Autodesk Inventor part; units mm, degrees
ref_plane "YZ Plane" through (0, 0, 0) normal (1, 0, 0) x (0, 1, 0)
ref_plane "XZ Plane" through (0, 0, 0) normal (0, 1, 0) x (-1, 0, 0)
ref_plane "XY Plane" through (0, 0, 0) normal (0, 0, 1) x (1, 0, 0)
sketch "Sketch1" plane through (0, 0, 0) normal (0, 0, 1) x (1, 0, 0)
  line L0 (0, 0) -> (457.2, 0)
  line L1 (457.2, 0) -> (457.2, 457.2)
  line L2 (457.2, 457.2) -> (0, 457.2)
  line L3 (0, 457.2) -> (0, 0)
  dimension "d0" = 457.2
  dimension "d1" = 457.2
extrude "Extrusion1" add sketch "Sketch1" along normal blind 25.4
sketch "Sketch2" plane through (0, 0, 0) normal (-1, 0, 0) x (0, 0, 1)
  line L0 (0, 457.2) -> (25.4, 457.2)
  line L1 (0, 457.2) -> (0, 304.8)
  line L2 (0, 0) -> (0, 457.2)
  line L3 (25.4, 0) -> (25.4, 457.2)
  line L4 (0, 304.8) -> (25.4, 457.2)
  dimension "d4" = 152.4
extrude "Extrusion2" cut sketch "Sketch2" against normal blind 457.2
sketch "Sketch3" plane through (0, 0, 0) normal (-1, 0, 0) x (0, 0, 1)
  line L0 (25.4, 457.2) -> (25.4, 0)
  line L1 (25.4, 457.2) -> (0, 457.2)
  line L2 (0, 304.8) -> (0, 0)
  line L3 (0, 457.2) -> (0, 304.8)
  line L4 (0, 304.8) -> (25.4, 457.2)
extrude "Extrusion3" add sketch "Sketch3" against normal blind 152.4
sketch "Sketch4" plane through (457.2, 0, 25.4) normal (1, 0, 0) x (0, 0, -1)
  line L0 (0, 0) -> (0, 457.2)
  line L1 (0, 457.2) -> (25.4, 457.2)
  line L2 (25.4, 304.8) -> (0, 457.2)
  line L3 (25.4, 457.2) -> (25.4, 304.8)
  line L4 (25.4, 304.8) -> (0, 457.2)
  point P0 (25.4, 0)
extrude "Extrusion4" add sketch "Sketch4" against normal blind 152.4
sketch "Sketch5" plane through (0, 0, 0) normal (0, -1, 0) x (1, 0, 0)
  line L0 (304.8, 25.4) -> (152.4, 25.4)
  line L1 (304.8, 25.4) -> (152.4, 25.4)
  line L2 (152.4, 25.4) -> (152.4, 0)
  line L3 (152.4, 0) -> (304.8, 0)
  line L4 (304.8, 0) -> (304.8, 25.4)
  point P0 (0, 0)
extrude "Extrusion5" cut sketch "Sketch5" against normal blind 304.8
properties part number "BackLiftProtoPart3"
For this review, take the finished solid that the model builds, in its own axes (mm). A direction names the side the tool comes from. Round coordinates to 2 decimals unless told otherwise and drop trailing zeros. Write each loop counter-clockwise with the first axis right and the second up, starting at its lowest first coordinate (ties: lowest second). Pieces come first, ordered by that corner, then holes.
1) Take a section at B-B on z = 7.25. Give the boundary of the cut face in (x, y).
Answer below:
outline: (0, 0) - (152.4, 0) - (152.4, 304.8) - (304.8, 304.8) - (304.8, 0) - (457.2, 0) - (457.2, 457.2) - (304.8, 457.2) - (304.8, 348.3) - (152.4, 348.3) - (152.4, 457.2) - (0, 457.2) - close
2) Take a section at A-A on y = 36.5. Give the boundary of the cut face in (x, z), then the cut area to 3 significant figures.
Answer below:
outline: (0, 0) - (152.4, 0) - (152.4, 25.4) - (0, 25.4) - close; (304.8, 0) - (457.2, 0) - (457.2, 25.4) - (304.8, 25.4) - close
area: 7,740 mm2
3) Machinability: for faces 1 (the face through (228, 304.8, 13)), 2 (the face through (227.53, 379.93, 12.52)), 3 (the face through (75, 0, 13)), which of the approach directions +Z, -Z, +X, -X, +Y, -Y give a long, thin tool a straight path to every point of the face, cutting with its end or side? Answer none if there is none.
Answer below:
face 1: +Z, -Z, -Y
face 2: -Z, +Y
face 3: +Z, -Z, +X, -X, -Y
4) Take a section at C-C on x = 172. Give the boundary of the cut face in (y, z).
Answer below:
outline: (304.8, 0) - (457.2, 25.4) - (304.8, 25.4) - close
5) Insertion check: pin 1 Ø12 at (y, z) = (197.5, 21.5) entering from -X; pin 2 Ø12.5 at (x, z) = (232.5, 17.5) entering from -Y. Each pin has a flat end and moves straight along its axis. Give the tip position at first contact, or say it passes through.
Answer below:
pin 1: stops at x = 0
pin 2: stops at y = 304.8
6) Mouldability with a two-part tool opening along X and no side actions: class faces 4 (the face through (457.2, 232, 13)), 5 (the face through (304.8, 150, 13)), 6 (the face through (382, 457.2, 13)) as +X half, -X half, draft (parallel to the pull), parting line (faces both ways), or undercut.
Answer below:
face 4: +X half
face 5: undercut
face 6: draft
7) Take a section at D-D on y = 339.5. Give the boundary of the cut face in (x, z), then the cut area to 3 significant figures.
Answer below:
outline: (0, 0) - (152.4, 0) - (152.4, 5.78) - (304.8, 5.78) - (304.8, 0) - (457.2, 0) - (457.2, 25.4) - (0, 25.4) - close
area: 10,700 mm2
8) For line 1 along X through (y, z) = (175, 6.25); line 2 along Z through (x, y) = (178.5, 435.5); line 3 along Z through (x, y) = (195, 310.5), list the stretches that pass through material, from the lowest coordinate up.
Answer below:
line 1: x = 0 to 152.4, 304.8 to 457.2
line 2: z = 21.78 to 25.4
line 3: z = 0.95 to 25.4
